The model under review builds one solid part; all positions refer to its coordinate system, in mm. A direction names the side the tool comes from. Round coordinates to 2 decimals unless told otherwise and drop trailing zeros. Loops run counter-clockwise (first coordinate to the right, second up) from the corner with the lowest first, then second, coordinate; pieces in that order, holes last. Notation, with made-up numbers: (76.25, -34.5) -> (95.25, -34.5) arc R25 cw to (95.25, -18.5) -> close; hole circle Ø3 at (75, 56.5). An arc over 180 degrees is marked (long way). Write each question's results on one line, items separated by ' | '. Start each with the question number.
Item 1: We need section B-B (z = -11). Give the boundary of the cut face in (x, y) (3 decimals).
Item 2: For L1, parallel to Y at x = 0, z = -18.75; L2, parallel to Z at x = 17, y = 17.5; L3, parallel to Z at x = 1, y = 17, list the stretches that pass through material, from the lowest coordinate up. Write a range as from..to.
Item 3: We need section A-A (y = 0). Give the boundary of the cut face in (x, z) (1 decimal).
Item 4: Clearance check with flat-ended pins moving along their axes: pin 1 Ø10.5 at (x, y) = (0, 0) entering from -Z; pin 2 Ø1.7 at (x, y) = (-15.5, -15.5) entering from +Z; pin 3 Ø3 at (x, z) = (-9.52, -18.48) entering from -Y. State where each tip first meets the part, or that it passes through.
Item 5: Tool access review of faces 1 (the cylindrical face through (10.754, 15.97, 16.876)), 2 (the cylindrical face through (0.69, -3.1, -11.18)), 3 (the cylindrical face through (-13.59, 14.48, 0.2)), 4 (the cylindrical face through (-16.73, -5.27, 24.06)), 5 (the flat face through (15, 15, 25.629)): name each direction out of +Z, -Z, +X, -X, +Y, -Y from which nothing blocks a thin tool from reaching the whole face with its end or side.
Item 6: We need section C-C (z = 5). Give the boundary of the cut face in (x, y).
Item 7: Mouldability with a two-part tool opening along Z and no side actions: class faces 6 (the flat face through (0, 0, 64.11)), 7 (the cylindrical face through (-7.554, 15.97, -18.916)), 8 (the cylindrical face through (-17.78, -15.95, 23.87)) as pulls with the +Z half, pulls with the -Z half, needs draft (parallel to the pull), parting line crosses it, or undercut.
Item 8: We need section D-D (x = 5). Give the boundary of the cut face in (y, z), and give its area (3 significant figures).
from build123d import *

# Parameters (mm, degrees)
SKETCH1_R                       = 18.4531
CAN_DEPTH                       = 14.5415
SKETCH2_W                       = 38.3032
SKETCH2_H                       = 38.2016
FRONT_FLANGE_DEPTH              = 7.62
SKETCH3_R                       = 17.5387
FRONT_BEARING_DEPTH             = 3.8481
SKETCH4_R                       = 6.3373
SHAFT_DEPTH                     = 38.1
KEYWAY_START                    = -35.814
KEYWAY_DEPTH                    = 35.814
SKETCH7_R                       = 2.794
SCREW_HEADS_DEPTH               = 3.4671
SKETCH8_R                       = 1.651
SCREW_THREADS_DEPTH             = 36.703
F_10_32_TAPPED_HOLE1_AT_2_COUNT = 2
F_10_32_TAPPED_HOLE1_AT_2_PITCH = 19.05
F_10_32_TAPPED_HOLE1_AT_3_COUNT = 2
F_10_32_TAPPED_HOLE1_AT_3_PITCH = 41.577906982
F_10_32_TAPPED_HOLE1_AT_4_COUNT = 2
F_10_32_TAPPED_HOLE1_AT_4_PITCH = 36.957
SKETCH12_R                      = 8.763
BACK_RECESS_DEPTH               = 6.35
SKETCH13_R                      = 3.175
PINION_RECESS_DEPTH             = 9.398
FLANGE_CHAMFERS_SIZE            = 3.175
KEYWAY_FILLET_R                 = 1.5875


with BuildPart() as part:
    # Sketch1 → Can (new, symmetric)
    with BuildSketch(Plane.XY):
        with Locations(Location((0, 0, 0), (0, 0, 180))):
            Circle(SKETCH1_R)
    extrude(amount=CAN_DEPTH, both=True)

    # Sketch2 → Front Flange (add)
    with BuildSketch(Plane.XY.offset(14.5415)):
        Rectangle(SKETCH2_W, SKETCH2_H)
    front_flange = extrude(amount=FRONT_FLANGE_DEPTH)

    # Sketch3 → Front Bearing (add)
    with BuildSketch(Plane.XY.offset(22.1615)):
        with Locations(Location((0, 0, 0), (0, 0, 180))):
            Circle(SKETCH3_R)
    extrude(amount=FRONT_BEARING_DEPTH)

    # Sketch4 → Shaft (add)
    with BuildSketch(Plane.XY.offset(26.0096)):
        with Locations(Location((0, 0, 0), (0, 0, 180))):
            Circle(SKETCH4_R)
    extrude(amount=SHAFT_DEPTH)

    # Sketch6 → Keyway (cut)
    with BuildSketch(Plane.XY.offset(64.1096).offset(KEYWAY_START)):
        with BuildLine():
            Line((-1.5875, 6.135243682), (-1.5875, 4.611243682))
            Line((-1.5875, 4.611243682), (1.5875, 4.611243682))
            Line((1.5875, 4.611243682), (1.5875, 6.135243682))
            ThreePointArc((1.5875, 6.135243682), (0, 6.3373), (-1.5875, 6.135243682))
        make_face()
    extrude(amount=KEYWAY_DEPTH, mode=Mode.SUBTRACT)

    # Back Flange: Front Flange across plane
    add(front_flange.mirror(Plane.XY))

    # Sketch7 → Screw Heads (add)
    with BuildSketch(Plane.XY.offset(22.1615)):
        with Locations(Location((15.113, 15.113, 0), (0, 0, 180))):
            Circle(SKETCH7_R)
        with Locations(Location((-15.113, 15.113, 0), (0, 0, 180))):
            Circle(SKETCH7_R)
        with Locations(Location((-15.113, -15.113, 0), (0, 0, 180))):
            Circle(SKETCH7_R)
        with Locations(Location((15.113, -15.113, 0), (0, 0, 180))):
            Circle(SKETCH7_R)
    extrude(amount=SCREW_HEADS_DEPTH)

    # Sketch8 → Screw Threads (add)
    with BuildSketch(Plane.XY.offset(22.1615)):
        with Locations((-15.113, 15.113)):
            Circle(SKETCH8_R)
        with Locations((15.113, 15.113)):
            Circle(SKETCH8_R)
        with Locations((15.113, -15.113)):
            Circle(SKETCH8_R)
        with Locations((-15.113, -15.113)):
            Circle(SKETCH8_R)
    extrude(amount=-SCREW_THREADS_DEPTH)

    # Sketch10 → #10-32 Tapped Hole1 (revolve, cut)
    with BuildSketch(Plane(origin=(-9.525, 19.1008, 18.4785), x_dir=(0, 0, 1), z_dir=(1, 0, 0))):
        Polygon((0, 0), (0, 7.563317848), (2.0193, 6.35), (2.0193, 0), align=None)
    f_10_32_tapped_hole1 = revolve(axis=Axis((-9.525, 25.4508, 18.4785), (0, -1, 0)), mode=Mode.SUBTRACT)

    # #10-32 Tapped Hole1 at 2: #10-32 Tapped Hole1 ×2
    with Locations(*[(i * F_10_32_TAPPED_HOLE1_AT_2_PITCH, 0, 0) for i in range(1, F_10_32_TAPPED_HOLE1_AT_2_COUNT)]):
        add(f_10_32_tapped_hole1, mode=Mode.SUBTRACT)

    # #10-32 Tapped Hole1 at 3: #10-32 Tapped Hole1 ×2
    with Locations(*[Vector(0.4581760214209039, 0, -0.8888614815565536) * (i * F_10_32_TAPPED_HOLE1_AT_3_PITCH) for i in range(1, F_10_32_TAPPED_HOLE1_AT_3_COUNT)]):
        add(f_10_32_tapped_hole1, mode=Mode.SUBTRACT)

    # #10-32 Tapped Hole1 at 4: #10-32 Tapped Hole1 ×2
    with Locations(*[(0, 0, -i * F_10_32_TAPPED_HOLE1_AT_4_PITCH) for i in range(1, F_10_32_TAPPED_HOLE1_AT_4_COUNT)]):
        add(f_10_32_tapped_hole1, mode=Mode.SUBTRACT)

    # #10-32 Tapped Hole2: #10-32 Tapped Hole1 across plane
    add(f_10_32_tapped_hole1.mirror(Plane.ZX), mode=Mode.SUBTRACT)

    # #10-32 Tapped Hole2 copy 1 sketch → #10-32 Tapped Hole2 copy 1 (revolve, cut)
    with BuildSketch(Plane(origin=(9.525, -19.1008, 18.4785), x_dir=(0, 0, 1), z_dir=(1, 0, 0))):
        Polygon((0, 0), (0, -7.563317848), (2.0193, -6.35), (2.0193, 0), align=None)
    revolve(axis=Axis((9.525, -25.4508, 18.4785), (0, -1, 0)), mode=Mode.SUBTRACT)

    # #10-32 Tapped Hole2 copy 2 sketch → #10-32 Tapped Hole2 copy 2 (revolve, cut)
    with BuildSketch(Plane(origin=(9.525, -19.1008, -18.4785), x_dir=(0, 0, 1), z_dir=(1, 0, 0))):
        Polygon((0, 0), (0, -7.563317848), (2.0193, -6.35), (2.0193, 0), align=None)
    revolve(axis=Axis((9.525, -25.4508, -18.4785), (0, -1, 0)), mode=Mode.SUBTRACT)

    # #10-32 Tapped Hole2 copy 3 sketch → #10-32 Tapped Hole2 copy 3 (revolve, cut)
    with BuildSketch(Plane(origin=(-9.525, -19.1008, -18.4785), x_dir=(0, 0, 1), z_dir=(1, 0, 0))):
        Polygon((0, 0), (0, -7.563317848), (2.0193, -6.35), (2.0193, 0), align=None)
    revolve(axis=Axis((-9.525, -25.4508, -18.4785), (0, -1, 0)), mode=Mode.SUBTRACT)

    # Sketch12 → Back Recess (cut)
    with BuildSketch(Plane(origin=(0, 0, -22.1615), x_dir=(-1, 0, 0), z_dir=(0, 0, -1))):
        Circle(SKETCH12_R)
    extrude(amount=-BACK_RECESS_DEPTH, mode=Mode.SUBTRACT)

    # Sketch13 → Pinion Recess (cut)
    with BuildSketch(Plane(origin=(0, 0, -15.8115), x_dir=(-1, 0, 0), z_dir=(0, 0, -1))):
        Circle(SKETCH13_R)
    extrude(amount=-PINION_RECESS_DEPTH, mode=Mode.SUBTRACT)

    # Flange Chamfers
    flange_chamfers_edges = [part.edges().sort_by_distance(p)[0] for p in [
        (19.1516, 19.1008, -18.3515),
        (19.1516, -19.1008, -18.3515),
        (-19.1516, -19.1008, -18.3515),
        (-19.1516, 19.1008, -18.3515),
        (19.1516, -19.1008, 18.3515),
        (19.1516, 19.1008, 18.3515),
        (-19.1516, 19.1008, 18.3515),
        (-19.1516, -19.1008, 18.3515),
    ]]
    chamfer(flange_chamfers_edges, length=FLANGE_CHAMFERS_SIZE)

    # Keyway Fillet
    keyway_fillet_edges = [part.edges().sort_by_distance(p)[0] for p in [
        (-1.5875, 5.373243682, 28.2956),
        (1.5875, 5.373243682, 28.2956),
    ]]
    fillet(keyway_fillet_edges, radius=KEYWAY_FILLET_R - 0.0001)  # a hair under: the kernel refuses the full size


solid = part.part
Here are the results:
1) outline: circle Ø36.906 at (0, 0); circle Ø3.302 at (-15.113, -15.113); circle Ø3.302 at (-15.113, 15.113); circle Ø3.302 at (15.113, -15.113); circle Ø3.302 at (15.113, 15.113); hole circle Ø6.35 at (0, 0)
2) L1: y = -19.1..-8.76, 8.76..19.1 | L2: z = -22.16..-14.54, 14.54..22.16 | L3: z = -22.16..26.01
3) outline: (-19.2, -22.2) -> (-8.8, -22.2) -> (-8.8, -15.8) -> (-3.2, -15.8) -> (-3.2, -6.4) -> (3.2, -6.4) -> (3.2, -15.8) -> (8.8, -15.8) -> (8.8, -22.2) -> (19.2, -22.2) -> (19.2, -14.5) -> (18.5, -14.5) -> (18.5, 14.5) -> (19.2, 14.5) -> (19.2, 22.2) -> (17.5, 22.2) -> (17.5, 26) -> (6.3, 26) -> (6.3, 64.1) -> (-6.3, 64.1) -> (-6.3, 26) -> (-17.5, 26) -> (-17.5, 22.2) -> (-19.2, 22.2) -> (-19.2, 14.5) -> (-18.5, 14.5) -> (-18.5, -14.5) -> (-19.2, -14.5) -> close
4) pin 1: stops at z = -15.81 | pin 2: stops at z = 25.63 | pin 3: stops at y = -12.44
5) face 1: +Y | face 2: -Z | face 3: none | face 4: +Z | face 5: +Z, +X, +Y
6) outline: circle Ø36.91 at (0, 0); circle Ø3.3 at (-15.11, -15.11); circle Ø3.3 at (-15.11, 15.11); circle Ø3.3 at (15.11, -15.11); circle Ø3.3 at (15.11, 15.11)
7) face 6: pulls with the +Z half | face 7: undercut | face 8: needs draft
8) outline: (-19.1, -22.16) -> (-7.2, -22.16) -> (-7.2, -15.81) -> (7.2, -15.81) -> (7.2, -22.16) -> (19.1, -22.16) -> (19.1, -14.54) -> (17.76, -14.54) -> (17.76, 14.54) -> (19.1, 14.54) -> (19.1, 22.16) -> (16.81, 22.16) -> (16.81, 26.01) -> (3.89, 26.01) -> (3.89, 64.11) -> (-3.89, 64.11) -> (-3.89, 26.01) -> (-16.81, 26.01) -> (-16.81, 22.16) -> (-19.1, 22.16) -> (-19.1, 14.54) -> (-17.76, 14.54) -> (-17.76, -14.54) -> (-19.1, -14.54) -> close | area: 1,950 mm2
